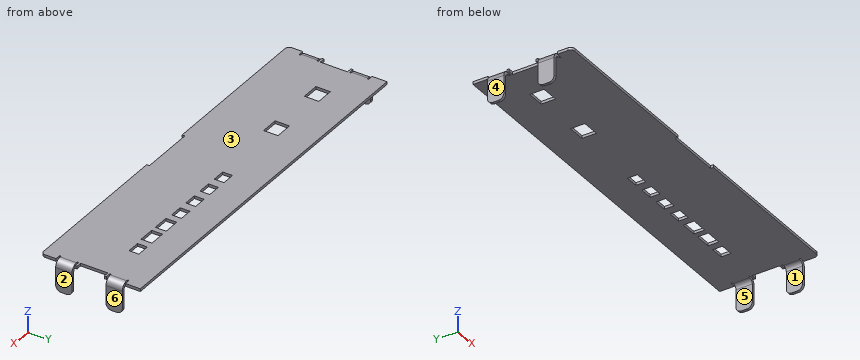
```python
from build123d import *

# Parameters (mm, degrees)
SKETCH1_W                       = 139
SKETCH1_H                       = 36.5
BASE_FLANGE1_DEPTH              = 1
EDGE_FLANGE1_STRIP_W            = 7
EDGE_FLANGE1_STRIP_H            = 1
EDGE_FLANGE1_STRIP_CUT_DEPTH    = 6
EDGE_FLANGE1_RELIEF_W           = 7.5
EDGE_FLANGE1_RELIEF_H           = 0.5
EDGE_FLANGE1_RELIEF_CUT_DEPTH   = 1
EDGE_FLANGE1_STRIP_2_W          = 7
EDGE_FLANGE1_STRIP_2_H          = 1
EDGE_FLANGE1_STRIP_CUT_2_DEPTH  = 6
EDGE_FLANGE1_RELIEF_2_W         = 7.5
EDGE_FLANGE1_RELIEF_2_H         = 0.5
EDGE_FLANGE1_RELIEF_CUT_2_DEPTH = 1
EDGE_FLANGE1_DEPTH              = 6
EDGE_FLANGE1_START              = -1
EDGE_FLANGE1_FLAT_DEPTH         = 1
EDGE_FLANGE1_BEND_DEPTH         = 6
EDGE_FLANGE1_FLAT_2_DEPTH       = 1
EDGE_FLANGE2_STRIP_W            = 7
EDGE_FLANGE2_STRIP_H            = 1
EDGE_FLANGE2_STRIP_CUT_DEPTH    = 6
EDGE_FLANGE2_RELIEF_W           = 7.5
EDGE_FLANGE2_RELIEF_H           = 0.5
EDGE_FLANGE2_RELIEF_CUT_DEPTH   = 1
EDGE_FLANGE2_STRIP_2_W          = 7
EDGE_FLANGE2_STRIP_2_H          = 1
EDGE_FLANGE2_STRIP_CUT_2_DEPTH  = 6
EDGE_FLANGE2_RELIEF_2_W         = 7.5
EDGE_FLANGE2_RELIEF_2_H         = 0.5
EDGE_FLANGE2_RELIEF_CUT_2_DEPTH = 1
EDGE_FLANGE2_DEPTH              = 6
EDGE_FLANGE2_START              = 1
EDGE_FLANGE2_FLAT_DEPTH         = 1
EDGE_FLANGE2_BEND_DEPTH         = 6
EDGE_FLANGE2_FLAT_2_DEPTH       = 1
SKETCH20_W                      = 20
SKETCH20_H                      = 1
SKETCH20_W_2                    = 2
SKETCH20_H_2                    = 10
CUT_EXTRUDE1_DEPTH              = 10
FILLET1_R                       = 1.5
SKETCH28_W                      = 4.80000148
SKETCH28_H                      = 3.5999988
SKETCH28_H_2                    = 3.597941299
SKETCH28_W_2                    = 5.99999908
SKETCH28_H_3                    = 4.00000054
SKETCH28_W_3                    = 6.50000116
SKETCH28_H_4                    = 5.30000102
CUT_EXTRUDE3_DEPTH              = 10


# Sheet-metal steps are written as plain solids
with BuildPart() as part:
    # Sketch1 → Base-Flange1 (new body)
    with BuildSketch(Plane.XY):
        with Locations((0.929014267, 0)):
            Rectangle(SKETCH1_W, SKETCH1_H)
    extrude(amount=-BASE_FLANGE1_DEPTH)

    # Edge-Flange1 strip (across the edge) → Edge-Flange1 strip cut (cut)
    with BuildSketch(Plane(origin=(-68.570985733, 6.25, -1), x_dir=(1, 0, 0), z_dir=(0, 1, 0))):
        with Locations((-2, -0.5)):
            Rectangle(EDGE_FLANGE1_STRIP_W, EDGE_FLANGE1_STRIP_H)
    extrude(amount=EDGE_FLANGE1_STRIP_CUT_DEPTH, mode=Mode.SUBTRACT)

    # Edge-Flange1 relief (on the sheet) → Edge-Flange1 relief cut (cut)
    with BuildSketch(Plane(origin=(-67.070985733, 6.25, -1), x_dir=(1, 0, 0), z_dir=(0, 0, -1))):
        with Locations((-3.25, 0.25)):
            Rectangle(EDGE_FLANGE1_RELIEF_W, EDGE_FLANGE1_RELIEF_H)
        with Locations((-3.25, -6.25)):
            Rectangle(EDGE_FLANGE1_RELIEF_W, EDGE_FLANGE1_RELIEF_H)
    extrude(amount=-EDGE_FLANGE1_RELIEF_CUT_DEPTH, mode=Mode.SUBTRACT)

    # Edge-Flange1 strip 2 (across the edge) → Edge-Flange1 strip cut 2 (cut)
    with BuildSketch(Plane(origin=(70.429014267, 12.25, -1), x_dir=(-1, 0, 0), z_dir=(0, -1, 0))):
        with Locations((-2, -0.5)):
            Rectangle(EDGE_FLANGE1_STRIP_2_W, EDGE_FLANGE1_STRIP_2_H)
    extrude(amount=EDGE_FLANGE1_STRIP_CUT_2_DEPTH, mode=Mode.SUBTRACT)

    # Edge-Flange1 relief 2 (on the sheet) → Edge-Flange1 relief cut 2 (cut)
    with BuildSketch(Plane(origin=(68.929014267, 12.25, -1), x_dir=(-1, 0, 0), z_dir=(0, 0, -1))):
        with Locations((-3.25, 0.25)):
            Rectangle(EDGE_FLANGE1_RELIEF_2_W, EDGE_FLANGE1_RELIEF_2_H)
        with Locations((-3.25, -6.25)):
            Rectangle(EDGE_FLANGE1_RELIEF_2_W, EDGE_FLANGE1_RELIEF_2_H)
    extrude(amount=-EDGE_FLANGE1_RELIEF_CUT_2_DEPTH, mode=Mode.SUBTRACT)

    # Edge-Flange1 bend section (across the edge) → Edge-Flange1 (add)
    with BuildSketch(Plane(origin=(-68.570985733, 6.25, -1), x_dir=(1, 0, 0), z_dir=(0, 1, 0))):
        with BuildLine():
            Line((-1, 1.5), (0, 1.5))
            ThreePointArc((0, 1.5), (0.439339828, 0.439339828), (1.5, 0))
            Line((1.5, 0), (1.5, -1))
            ThreePointArc((1.5, -1), (-0.267766953, -0.267766953), (-1, 1.5))
        make_face()
    extrude(amount=EDGE_FLANGE1_DEPTH)

    # Edge-Flange1 profile (on flange) → Edge-Flange1 flat (add)
    with BuildSketch(Plane(origin=(-68.570985733, 0, -1), x_dir=(0, -1, 0), z_dir=(1, 0, 0)).offset(EDGE_FLANGE1_START)):
        with BuildLine():
            ThreePointArc((-6.25, 8), (-6.835786438, 9.414213562), (-8.25, 10))
            Line((-8.25, 10), (-10.25, 10))
            ThreePointArc((-10.25, 10), (-11.664213562, 9.414213562), (-12.25, 8))
            Line((-12.25, 8), (-12.25, 1.5))
            Line((-12.25, 1.5), (-6.25, 1.5))
            Line((-6.25, 1.5), (-6.25, 8))
        make_face()
    extrude(amount=EDGE_FLANGE1_FLAT_DEPTH)

    # Edge-Flange1 bend section 2 (across the edge) → Edge-Flange1 bend (add)
    with BuildSketch(Plane(origin=(70.429014267, 12.25, -1), x_dir=(-1, 0, 0), z_dir=(0, -1, 0))):
        with BuildLine():
            Line((-1, 1.5), (0, 1.5))
            ThreePointArc((0, 1.5), (0.439339828, 0.439339828), (1.5, 0))
            Line((1.5, 0), (1.5, -1))
            ThreePointArc((1.5, -1), (-0.267766953, -0.267766953), (-1, 1.5))
        make_face()
    extrude(amount=EDGE_FLANGE1_BEND_DEPTH)

    # Edge-Flange1 profile 2 (on flange) → Edge-Flange1 flat 2 (add)
    with BuildSketch(Plane(origin=(70.429014267, 0, -1), x_dir=(0, 1, 0), z_dir=(-1, 0, 0)).offset(EDGE_FLANGE1_START)):
        with BuildLine():
            Line((12.25, 1.5), (12.25, 8))
            ThreePointArc((12.25, 8), (11.664213562, 9.414213562), (10.25, 10))
            Line((10.25, 10), (8.25, 10))
            ThreePointArc((8.25, 10), (6.835786438, 9.414213562), (6.25, 8))
            Line((6.25, 8), (6.25, 1.5))
            Line((6.25, 1.5), (12.25, 1.5))
        make_face()
    extrude(amount=EDGE_FLANGE1_FLAT_2_DEPTH)

    # Edge-Flange2 strip (across the edge) → Edge-Flange2 strip cut (cut)
    with BuildSketch(Plane(origin=(70.429014267, -6.25, -1), x_dir=(-1, 0, 0), z_dir=(0, -1, 0))):
        with Locations((-2, -0.5)):
            Rectangle(EDGE_FLANGE2_STRIP_W, EDGE_FLANGE2_STRIP_H)
    extrude(amount=EDGE_FLANGE2_STRIP_CUT_DEPTH, mode=Mode.SUBTRACT)

    # Edge-Flange2 relief (on the sheet) → Edge-Flange2 relief cut (cut)
    with BuildSketch(Plane(origin=(68.929014267, -6.25, -1), x_dir=(-1, 0, 0), z_dir=(0, 0, -1))):
        with Locations((-3.25, 0.25)):
            Rectangle(EDGE_FLANGE2_RELIEF_W, EDGE_FLANGE2_RELIEF_H)
        with Locations((-3.25, -6.25)):
            Rectangle(EDGE_FLANGE2_RELIEF_W, EDGE_FLANGE2_RELIEF_H)
    extrude(amount=-EDGE_FLANGE2_RELIEF_CUT_DEPTH, mode=Mode.SUBTRACT)

    # Edge-Flange2 strip 2 (across the edge) → Edge-Flange2 strip cut 2 (cut)
    with BuildSketch(Plane(origin=(-68.570985733, -12.25, -1), x_dir=(1, 0, 0), z_dir=(0, 1, 0))):
        with Locations((-2, -0.5)):
            Rectangle(EDGE_FLANGE2_STRIP_2_W, EDGE_FLANGE2_STRIP_2_H)
    extrude(amount=EDGE_FLANGE2_STRIP_CUT_2_DEPTH, mode=Mode.SUBTRACT)

    # Edge-Flange2 relief 2 (on the sheet) → Edge-Flange2 relief cut 2 (cut)
    with BuildSketch(Plane(origin=(-67.070985733, -12.25, -1), x_dir=(1, 0, 0), z_dir=(0, 0, -1))):
        with Locations((-3.25, 0.25)):
            Rectangle(EDGE_FLANGE2_RELIEF_2_W, EDGE_FLANGE2_RELIEF_2_H)
        with Locations((-3.25, -6.25)):
            Rectangle(EDGE_FLANGE2_RELIEF_2_W, EDGE_FLANGE2_RELIEF_2_H)
    extrude(amount=-EDGE_FLANGE2_RELIEF_CUT_2_DEPTH, mode=Mode.SUBTRACT)

    # Edge-Flange2 bend section (across the edge) → Edge-Flange2 (add)
    with BuildSketch(Plane(origin=(70.429014267, -6.25, -1), x_dir=(-1, 0, 0), z_dir=(0, -1, 0))):
        with BuildLine():
            Line((-1, 1.5), (0, 1.5))
            ThreePointArc((0, 1.5), (0.439339828, 0.439339828), (1.5, 0))
            Line((1.5, 0), (1.5, -1))
            ThreePointArc((1.5, -1), (-0.267766953, -0.267766953), (-1, 1.5))
        make_face()
    extrude(amount=EDGE_FLANGE2_DEPTH)

    # Edge-Flange2 profile (on flange) → Edge-Flange2 flat (add)
    with BuildSketch(Plane(origin=(70.429014267, 0, -1), x_dir=(0, -1, 0), z_dir=(1, 0, 0)).offset(EDGE_FLANGE2_START)):
        with BuildLine():
            Line((12.25, 1.5), (12.25, 8))
            ThreePointArc((12.25, 8), (11.664213562, 9.414213562), (10.25, 10))
            Line((10.25, 10), (8.25, 10))
            ThreePointArc((8.25, 10), (6.835786438, 9.414213562), (6.25, 8))
            Line((6.25, 8), (6.25, 1.5))
            Line((6.25, 1.5), (12.25, 1.5))
        make_face()
    extrude(amount=-EDGE_FLANGE2_FLAT_DEPTH)

    # Edge-Flange2 bend section 2 (across the edge) → Edge-Flange2 bend (add)
    with BuildSketch(Plane(origin=(-68.570985733, -12.25, -1), x_dir=(1, 0, 0), z_dir=(0, 1, 0))):
        with BuildLine():
            Line((-1, 1.5), (0, 1.5))
            ThreePointArc((0, 1.5), (0.439339828, 0.439339828), (1.5, 0))
            Line((1.5, 0), (1.5, -1))
            ThreePointArc((1.5, -1), (-0.267766953, -0.267766953), (-1, 1.5))
        make_face()
    extrude(amount=EDGE_FLANGE2_BEND_DEPTH)

    # Edge-Flange2 profile 2 (on flange) → Edge-Flange2 flat 2 (add)
    with BuildSketch(Plane(origin=(-68.570985733, 0, -1), x_dir=(0, 1, 0), z_dir=(-1, 0, 0)).offset(EDGE_FLANGE2_START)):
        with BuildLine():
            ThreePointArc((-6.25, 8), (-6.835786438, 9.414213562), (-8.25, 10))
            Line((-8.25, 10), (-10.25, 10))
            ThreePointArc((-10.25, 10), (-11.664213562, 9.414213562), (-12.25, 8))
            Line((-12.25, 8), (-12.25, 1.5))
            Line((-12.25, 1.5), (-6.25, 1.5))
            Line((-6.25, 1.5), (-6.25, 8))
        make_face()
    extrude(amount=-EDGE_FLANGE2_FLAT_2_DEPTH)

    # Sketch20 → Cut-Extrude1 (cut)
    with BuildSketch(Plane(origin=(0, 0, -1), x_dir=(-1, 0, 0), z_dir=(0, 0, -1))):
        with Locations((-0.929014267, -17.75)):
            Rectangle(SKETCH20_W, SKETCH20_H)
        with Locations((-69.429014267, 0)):
            Rectangle(SKETCH20_W_2, SKETCH20_H_2)
        with Locations((67.570985733, 0)):
            Rectangle(SKETCH20_W_2, SKETCH20_H_2)
    extrude(amount=-CUT_EXTRUDE1_DEPTH, mode=Mode.SUBTRACT)

    # Fillet1
    fillet1_edges = [part.edges().sort_by_distance(p)[0] for p in [
        (70.429014267, -18.25, -0.5),
        (-68.570985733, -18.25, -0.5),
    ]]
    fillet(fillet1_edges, radius=FILLET1_R)

    # Sketch28 → Cut-Extrude3 (cut)
    with BuildSketch(Plane.XY):
        with Locations((3.972975907, 5.4002406)):
            Rectangle(SKETCH28_W, SKETCH28_H)
        with Locations((11.972975147, 5.4002406)):
            Rectangle(SKETCH28_W, SKETCH28_H)
        with Locations((19.972974387, 5.4002406)):
            Rectangle(SKETCH28_W, SKETCH28_H)
        with Locations((27.972973627, 5.39921185)):
            Rectangle(SKETCH28_W, SKETCH28_H_2)
        with Locations((35.972972867, 5.20023973)):
            Rectangle(SKETCH28_W_2, SKETCH28_H_3)
        with Locations((43.972972107, 5.20023973)):
            Rectangle(SKETCH28_W_2, SKETCH28_H_3)
        with Locations((51.972971347, 5.4002406)):
            Rectangle(SKETCH28_W, SKETCH28_H)
        with Locations((-51.082027013, 4.05023949)):
            Rectangle(SKETCH28_W_3, SKETCH28_H_4)
        with Locations((-28.082027293, 4.05023949)):
            Rectangle(SKETCH28_W_3, SKETCH28_H_4)
    extrude(amount=-CUT_EXTRUDE3_DEPTH, mode=Mode.SUBTRACT)


solid = part.part
```
The model under review builds one solid part; all positions refer to its coordinate system, in mm. Face numbers are marked on the shaded views. A direction names the side the tool comes from. Give positions to 0.01 mm unless a question says otherwise; leave off trailing zeros. Write each loop counter-clockwise with the first axis right and the second up, starting at its lowest first coordinate (ties: lowest second). Pieces come first, ordered by that corner, then holes. Notation, with made-up numbers: M 39,29.25 L 77,29.25 A12 ccw 77,46.25 Z; hole C -25.75,31 d8. An arc over 180 degrees is marked long. Answer in a Markdown table with one row per item.
Item 1: For line 1 along X through (y, z) = (-9.5, -5.25); line 2 along Z through (x, y) = (41, -4.5), list the stretches that pass through material, from the lowest coordinate up.
Check sheet entries:
| item | result |
|---|---|
| line 1 | -69.57 to -68.57, 70.43 to 71.43 |
| line 2 | -1 to 0 |
Item 2: Add section A-A on z = -5. Give the boundary of the cut face in (x, y), plus the area to 3 significant figures.
Check sheet entries:
| item | result |
|---|---|
| outline | M -69.57,-12.25 L -68.57,-12.25 L -68.57,-6.25 L -69.57,-6.25 Z; M -69.57,6.25 L -68.57,6.25 L -68.57,12.25 L -69.57,12.25 Z; M 70.43,-12.25 L 71.43,-12.25 L 71.43,-6.25 L 70.43,-6.25 Z; M 70.43,6.25 L 71.43,6.25 L 71.43,12.25 L 70.43,12.25 Z |
| area | 24.0 mm2 |
Item 3: Add section B-B on x = 27. Give the boundary of the cut face in (y, z), plus the area to 3 significant figures.
Check sheet entries:
| item | result |
|---|---|
| outline | M -18.25,-1 L 3.6,-1 L 3.6,0 L -18.25,0 Z; M 7.2,-1 L 18.25,-1 L 18.25,0 L 7.2,0 Z |
| area | 32.9 mm2 |
Item 4: Add section C-C on y = -1. Give the boundary of the cut face in (x, z).
Check sheet entries:
| item | result |
|---|---|
| outline | M -66.57,-1 L 68.43,-1 L 68.43,0 L -66.57,0 Z |
Item 5: Draft analysis for pull direction X (two halves, no side actions). For the marked faces 3, 4, 5 and 6, state which applies: +X half, -X half, draft (parallel to the pull), parting line (faces both ways), or undercut.
Check sheet entries:
| item | result |
|---|---|
| face 3 | draft |
| face 4 | -X half |
| face 5 | undercut |
| face 6 | +X half |
Item 6: Add section D-D on x = 58.5. Give the boundary of the cut face in (y, z).
Check sheet entries:
| item | result |
|---|---|
| outline | M -18.25,-1 L 18.25,-1 L 18.25,0 L -18.25,0 Z |
Item 7: Tool access review of the marked faces 1 and 2: name each direction out of +Z, -Z, +X, -X, +Y, -Y from which nothing blocks a thin tool from reaching the whole face with its end or side.
Check sheet entries:
| item | result |
|---|---|
| face 1 | -Z, +Y, -Y |
| face 2 | +Z, -Z, +X, +Y, -Y |
Item 8: For P1, Ø1.5, axis at x = -2.5, y = -4.5, coming from the -Z side; P2, Ø2.5, axis at x = -68.5, z = -4, coming from the -Y side; P3, Ø1.1, axis at y = 5.5, z = -0.5, coming from the +X side, all flat-tipped, find the tip position at first contact; note any pin that passes through.
Check sheet entries:
| item | result |
|---|---|
| P1 | z = -1 |
| P2 | y = -12.25 |
| P3 | x = 70.43 |
